Autodesk Fusion 360 part; units mm, degrees
sketch "Sketch1" plane through (0, 0, 0) normal (0, 0, 1) x (1, 0, 0)
  line L0 (0, 0) -> (62.725, 0)
  line L1 (0, 0) -> (-62.725, 0)
  line L2 (62.725, 0) -> (62.725, -15)
  circle A0 centre (-57.125, -5.6) radius 1.5
  line L3 (-62.725, 0) -> (-62.725, -15)
  line L4 (-62.725, -15) -> (62.725, -15)
  circle A1 centre (57.125, -5.6) radius 1.5
  line L5 (0, 0) -> (0, 109.7609) construction
  line L6 (-62.725, 0) -> (0, 109.7609)
  line L7 (62.725, 0) -> (0, 109.7609)
  line L8 (0, 109.7609) -> (0, 100)
  line L9 (0, 100) -> (-55, 0)
  line L10 (0, 100) -> (55, 0)
  circle A2 centre (-57.125, -5.6) radius 3.5
  circle A3 centre (57.125, -5.6) radius 3.5
  dimension "d1" = 62.725
  dimension "d2" = 62.725
  dimension "d3" = 15
  dimension "d8" = 3
  dimension "d9" = 15
  dimension "d12" = 3
  dimension "d33" = 2
  dimension "d34" = 2
extrude "Extrude1" add sketch "Sketch1" against normal blind 3 contours L0 L1 L2 L3 L4 | A2 | A3 makes body 1
extrude "Extrude2" add sketch "Sketch1" against normal blind 62 separate body contours L0 L7 L8 L10 | L1 L6 L8 L9 makes body 2
extrude "Extrude3" add sketch "Sketch1" against normal blind 3 contours L0 L1 L9 L10 bodies 1 2
sketch "Sketch2" plane through (0, 0, -62) normal (0, 0, -1) x (1, 0, 0)
  line L0 (0, -100) -> (-55, 0)
  line L1 (-55, 0) -> (-62.725, 0)
  line L2 (-62.725, 0) -> (0, -109.7609)
  line L3 (0, -109.7609) -> (62.725, 0)
  line L4 (55, 0) -> (0, -100)
  line L5 (0, 0) -> (-62.725, 0)
  line L6 (0, 0) -> (62.725, 0)
  line L7 (62.725, 0) -> (62.725, 15)
  line L8 (-62.725, 0) -> (-62.725, 15)
  line L9 (-62.725, 15) -> (62.725, 15)
  line L10 (62.725, 0) -> (55, 0)
  circle A0 centre (57.125, 5.6) radius 2.5
  circle A1 centre (-57.125, 5.6) radius 2.5
  dimension "d23" = 5
  dimension "d24" = 5.6
  dimension "d25" = 5.6
  dimension "d26" = 5
  dimension "d27" = 5.6
  dimension "d28" = 5.6
extrude "Extrude4" add sketch "Sketch2" against normal blind 3 separate body contours L1 L5 L6 L7 L8 L9 L10 | A0 | A1 makes body 3
extrude "Extrude5" add sketch "Sketch2" against normal blind 3 contours L0 L4 L5 L6 bodies 1 3
extrude "Extrude6" add sketch "Sketch2" against normal blind 6 contours A0 | A1 bodies 1
extrude "Extrude7" cut sketch "Sketch1" against normal blind 1 contours A2 | A3 bodies 1
chamfer "Chamfer1" distance 1 angle 45 1 edges at (0, -15, -3) on bodies 1
extrude "Extrude8" add sketch "Sketch1" along normal blind 40 contours L0 L7 L8 L10 | L1 L6 L8 L9 bodies 1
sketch "Sketch3" plane through (-47.2833, 27.021, 0) normal (-0.8682, 0.4962, 0) x (-0.4962, -0.8682, 0)
  line L0 (-95.2975, 40) -> (-95.2975, -62)
  line L1 (-95.2975, -62) -> (31.122, -62)
  line L2 (31.122, -62) -> (31.122, -59)
  line L3 (31.122, -59) -> (31.122, -3)
  line L4 (31.122, -3) -> (31.122, 0)
  line L5 (31.122, 0) -> (31.122, 40)
  line L6 (31.122, 40) -> (-95.2975, 40)
  line L7 (-87.0975, 29) -> (22.9025, 29) construction
  line L8 (22.9025, 29) -> (22.9025, -51) construction
  line L9 (22.9025, -51) -> (-87.0975, -51) construction
  line L10 (-87.0975, -51) -> (-87.0975, 29) construction
  line L11 (23.5025, -51.6) -> (-87.6975, -51.6) construction
  line L12 (-87.6975, -51.6) -> (-87.6975, 29.6) construction
  line L13 (-87.6975, 29.6) -> (23.5025, 29.6) construction
  line L14 (23.5025, 29.6) -> (23.5025, -51.6) construction
  line L15 (-54.0975, -4) -> (-10.0975, -4)
  line L16 (-10.0975, -4) -> (-10.0975, -18)
  line L17 (-10.0975, -18) -> (-54.0975, -18)
  line L18 (-54.0975, -18) -> (-54.0975, -4)
  line L19 (-87.2975, 29.2) -> (23.1025, 29.2)
  line L20 (23.1025, 29.2) -> (23.1025, -51.2)
  line L21 (23.1025, -51.2) -> (-87.2975, -51.2)
  line L22 (-87.2975, -51.2) -> (-87.2975, 29.2)
  line L23 (-41.0975, -4) -> (-41.0975, -18)
  line L24 (-23.0975, -4) -> (-23.0975, -18)
  line L25 (-23.0975, -18) -> (-41.0975, -18)
  line L26 (-23.0975, -4) -> (-41.0975, -4)
  dimension "d40" = 110
  dimension "d41" = 80
  dimension "d42" = 11
  dimension "d43" = 8.2
  dimension "d44" = -0.6
  dimension "d55" = 33
  dimension "d66" = -0.2
  dimension "d67" = 13
  dimension "d68" = 13
extrude "Extrude12" cut sketch "Sketch3" against normal blind 2 contours L19 L20 L21 L22 bodies 1
extrude "Extrude13" cut sketch "Sketch3" against normal blind 15 contours L15 L17 L23 L24 L25 L26 bodies 1
mirror "Mirror2" about plane through (0, 0, 0) normal (1, 0, 0) of "Extrude12", "Extrude13"
fillet "Fillet2" radius 2 5 edges at (31.3625, 54.8805, 40) (-31.3625, 54.8805, 40) (0, 109.7609, -11) (31.3625, 54.8805, -62) (-31.3625, 54.8805, -62) on bodies 1
fillet "Fillet2" radius 2 8 edges at (-27.5, 50, 40) (27.5, 50, 40) (-55, 0, 20) (-62.725, 0, 20) (55, 0, 20) (62.725, 0, 20) (-58.8625, 0, 40) (58.8625, 0, 40) on bodies 1
equation "d15 = -56 mm - 6 mm"
Input: part model. Units: mm. Frame: model coordinates. A direction names the side the tool comes from. Round coordinates to 2 decimals unless told otherwise and drop trailing zeros. Write each loop counter-clockwise with the first axis right and the second up, starting at its lowest first coordinate (ties: lowest second). Pieces come first, ordered by that corner, then holes.
1) Cut plane B-B (y = 29). Count the separate pieces of the cut face and the enclosed holes in it, then the cut area to 3 significant figures.
2) Cut plane A-A (z = -44). Return the cut outline in (x, y) (3 decimals).
3) Cut plane C-C (z = 17.5). Return the cut outline in (x, y).
4) Draft query along X for faces 4 (the flat face through (59, -6, -1)), 5 (the flat face through (-57, -6, -56)), 6 (the cylindrical face through (-30.466, 55.3, 39.399)), 7 (the flat face through (-23, 68, -18)). Return one class per face: pulls with the +X half, pulls with the -X half, needs draft (parallel to the pull), parting line crosses it, or undercut.
5) Ray query, L1, parallel to Z at x = 24, y = 23.5; L2, parallel to Z at x = 24, y = 60.5; L3, parallel to X at y = 22, z = 17.5. Return the intervals inside material, ascending.
6) Contact query for flat-ended pins moving along their axis: P1, Ø10, axis at y = 21.5, z = 24.5, coming from the +X side; P2, Ø1, axis at y = 61.5, z = 22, coming from the +X side; P3, Ø5, axis at x = -21.5, z = -3, coming from the +Y side. Output: stop coordinate, or through.
7) Reachability of faces 1 (the cylindrical face through (53.63, -5.45, -0.49)), 2 (the flat face through (30, 55, -51.2)), 3 (the flat face through (-58, 0, 19)) from +Z, -Z, +X, -X, +Y, -Y: full face, straight path, thin tool, end or side. Return the list, or none.
Geometry says:
1. separate pieces: 1
1. enclosed holes: 3
1. area: 1,540 mm2
2. outline: (-62.725, 0) - (-55, 0) - (0, 100) - (55, 0) - (62.725, 0) - (58.746, 6.963) - (57.01, 5.971) - (2.23, 101.821) - (3.966, 102.813) - (47.523, 26.601) - (1.736, 106.722) arc R2 ccw to (-1.736, 106.722) - (-47.523, 26.601) - (-3.966, 102.813) - (-2.23, 101.821) - (-57.01, 5.971) - (-58.746, 6.963) - close
3. outline: (-61.01, 2.99) arc R2 ccw to (-59.28, 0) - (-56.18, 0) arc R2 ccw to (-54.43, 1.04) - (0, 100) - (54.43, 1.04) arc R2 ccw to (56.18, 0) - (59.28, 0) arc R2 ccw to (61.01, 2.99) - (58.75, 6.96) - (57.01, 5.97) - (2.23, 101.82) - (3.97, 102.81) - (47.52, 26.6) - (1.74, 106.72) arc R2 ccw to (-1.74, 106.72) - (-47.52, 26.6) - (-3.97, 102.81) - (-2.23, 101.82) - (-57.01, 5.97) - (-58.75, 6.96) - close
4. face 4: undercut
4. face 5: needs draft
4. face 6: pulls with the -X half
4. face 7: undercut
5. L1: z = -62 to -59, -3 to 0
5. L2: z = -62 to -18, -4 to 40
5. L3: x = -47.85 to -42.9, 42.9 to 47.85
6. P1: stops at x = 51.41
6. P2: stops at x = 27.87
6. P3: stops at y = 76.51
7. face 1: +Z
7. face 2: none
7. face 3: +Z, +X, -X, -Y
